```python
from build123d import *

# Parameters (mm, degrees)
SKETCH1_R           = 8
BOSS_EXTRUDE1_DEPTH = 2.5
SKETCH2_R           = 9
BOSS_EXTRUDE2_DEPTH = 4.5
SKETCH3_R           = 8
BOSS_EXTRUDE3_DEPTH = 0.25
SKETCH4_R           = 10
BOSS_EXTRUDE4_DEPTH = 6
SKETCH5_W           = 5
SKETCH5_H           = 5
CUT_EXTRUDE1_DEPTH  = 5
CHAMFER1_SIZE       = 1
CHAMFER2_SIZE       = 0.75


with BuildPart() as part:
    # Sketch1 → Boss-Extrude1 (new body)
    with BuildSketch(Plane.XY):
        Circle(SKETCH1_R)
    extrude(amount=BOSS_EXTRUDE1_DEPTH)

    # Sketch2 → Boss-Extrude2 (add)
    with BuildSketch(Plane.XY.offset(2.5)):
        Circle(SKETCH2_R)
    extrude(amount=BOSS_EXTRUDE2_DEPTH)

    # Sketch3 → Boss-Extrude3 (add)
    with BuildSketch(Plane.XY.offset(7)):
        Circle(SKETCH3_R)
    extrude(amount=BOSS_EXTRUDE3_DEPTH)

    # Sketch4 → Boss-Extrude4 (add)
    with BuildSketch(Plane.XY.offset(7.25)):
        Circle(SKETCH4_R)
    extrude(amount=BOSS_EXTRUDE4_DEPTH)

    # Sketch5 → Cut-Extrude1 (cut)
    with BuildSketch(Plane(origin=(0, 0, 0), x_dir=(-1, 0, 0), z_dir=(0, 0, -1))):
        Rectangle(SKETCH5_W, SKETCH5_H)
    extrude(amount=-CUT_EXTRUDE1_DEPTH, mode=Mode.SUBTRACT)

    # Chamfer1
    chamfer1_edges = [part.edges().sort_by_distance(p)[0] for p in [
        (-8, 0, 0),
    ]]
    chamfer(chamfer1_edges, length=CHAMFER1_SIZE)

    # Chamfer2
    chamfer2_edges = [part.edges().sort_by_distance(p)[0] for p in [
        (-10, 0, 13.25),
    ]]
    chamfer(chamfer2_edges, length=CHAMFER2_SIZE)


solid = part.part
```
Source: CAD feature listing. Evaluate the final solid. Frame: model axes, mm. A direction names the side the tool comes from. Give positions to 0.01 mm unless a question says otherwise; leave off trailing zeros. Loops run counter-clockwise (first coordinate to the right, second up) from the corner with the lowest first, then second, coordinate; pieces in that order, holes last. Notation, with made-up numbers: (-14, -10) -> (-1, -10) arc R24 ccw to (-1, 19) -> close; hole circle Ø11 at (-6, 37). An arc over 180 degrees is marked (long way). Use a Markdown table: item, result. Add a question column.
(1) Pull-direction query (Y, two-part tool) for faces 1 (the face through (-1.73, -7.81, 1.74)), 2 (the face through (0, 2.5, 2)), 3 (the face through (0, 0, 13.25)); classes: +Y half, -Y half, draft (parallel to the pull), parting line (faces both ways), or undercut.
(2) Section query B-B (z = 3.25). Output: boundary loops of the cut face in (x, y).
(3) Ray query, line 1 (Y direction, x = -1.75, z = 3); line 2 (Z direction, x = -4.75, y = -8.25); line 3 (Y direction, x = 6.75, z = 10). Return the intervals inside material, ascending.
(4) Section query A-A (x = 0). Output: boundary loops of the cut face in (y, z), then the cut area to 3 significant figures.
(5) Section query D-D (z = 7.75). Output: boundary loops of the cut face in (x, y).
(6) First-contact query: pin 1 Ø5.5 at (x, z) = (1, 3.5) entering from -Y; pin 2 Ø1.5 at (y, z) = (0.5, 3) entering from -X; pin 3 Ø1.5 at (x, y) = (0.5, -1) entering from -Z. Flat tips, straight axial feed; report the tip coordinate or a pass-through.
(7) Access query for faces 4 (the face through (-2.5, 0, 2)), 5 (the face through (-2.17, -9.76, 9.84)), 6 (the face through (0, 8.2, 7.25)). Directions: +Z, -Z, +X, -X, +Y, -Y. A direction counts if a zero-diameter tool reaches every point of the face in a straight line with its end or side. Return the directions, or none.
Checked values:
| question | item | result |
|---|---|---|
| 1 | face 1 | parting line |
| 1 | face 2 | undercut |
| 1 | face 3 | draft |
| 2 | outline | circle Ø18 at (0, 0); hole (-2.5, -2.5) -> (2.5, -2.5) -> (2.5, 2.5) -> (-2.5, 2.5) -> close |
| 3 | line 1 | -8.83 to -2.5, 2.5 to 8.83 |
| 3 | line 2 | 7.25 to 12.98 |
| 3 | line 3 | -7.38 to 7.38 |
| 4 | outline | (-10, 7.25) -> (-8, 7.25) -> (-8, 7) -> (-9, 7) -> (-9, 2.5) -> (-8, 2.5) -> (-8, 1) -> (-7, 0) -> (-2.5, 0) -> (-2.5, 5) -> (2.5, 5) -> (2.5, 0) -> (7, 0) -> (8, 1) -> (8, 2.5) -> (9, 2.5) -> (9, 7) -> (8, 7) -> (8, 7.25) -> (10, 7.25) -> (10, 12.5) -> (9.25, 13.25) -> (-9.25, 13.25) -> (-10, 12.5) -> close |
| 4 | area | 218 mm^2 |
| 5 | outline | circle Ø20 at (0, 0) |
| 6 | pin 1 | y = -9 |
| 6 | pin 2 | x = -9 |
| 6 | pin 3 | z = 5 |
| 7 | face 4 | -Z |
| 7 | face 5 | +Z, -Z |
| 7 | face 6 | none |
